Autodesk Inventor part; units mm, degrees
ref_plane "Work Plane1" through (13.4, 0, 0) normal (1, 0, 0) x (0, 1, 0)
ref_plane "XZ Plane" through (0, 0, 0) normal (0, 1, 0) x (-1, 0, 0)
ref_plane "XY Plane" through (0, 0, 0) normal (0, 0, 1) x (1, 0, 0)
sketch "Sketch1" plane through (0, 0, 0) normal (0, 0, 1) x (1, 0, 0)
  circle A0 centre (0, 0) radius 13.4
  circle A1 centre (0, 0) radius 11.75
  dimension "d0" = 26.8
  dimension "d3" = 23.5
extrude "Extrusion1" add sketch "Sketch1" along normal blind 300
ref_plane "Work Plane1" through (13.4, 0, 0) normal (1, 0, 0) x (0, 1, 0)
sketch "Sketch2" plane through (13.4, 0, 0) normal (1, 0, 0) x (0, 1, 0)
  circle A0 centre (0, 30) radius 4
  line L0 (0, -60) -> (0, 360)
  line L1 (13.4, 0) -> (-13.4, 0)
  circle A1 centre (0, 270) radius 4
  line L2 (13.4, 300) -> (-13.4, 300)
  point P0 (0, 0)
  dimension "d4" = 8
  dimension "d5" = 30
  dimension "d6" = 8
  dimension "d7" = 30
extrude "Extrusion2" cut sketch "Sketch2" against normal through all
equation "\"d0\" = PVC_out"
equation "\"d3\" = PVC_in"
equation "\"PVC_out\" = 26.8"
equation "\"PVC_in\" = 23.5"
properties part number "Steering PVC" material "PVC-Piping"
Source: CAD feature listing. Evaluate the final solid. Frame: model axes, mm. Coordinates: 2 decimals unless noted, no trailing zeros. Order: outer loops, then holes, each group sorted by start corner. A loop starts at its lowest first (then second) coordinate and runs counter-clockwise, first axis right, second up.
Item 1: Cut plane A-A (x = 0). Return loops of the section in (y, z), plus the area to 3 significant figures.
Output values:
outline: (-13.4, 0) - (-11.75, 0) - (-11.75, 300) - (-13.4, 300) - close; (11.75, 0) - (13.4, 0) - (13.4, 300) - (11.75, 300) - close
area: 990 mm2
Item 2: Material intervals for line 1 (Z direction, x = 12, y = 0); line 2 (Y direction, x = 0, z = 160); line 3 (Y direction, x = -11.8, z = 270), sorted ascending.
Output values:
line 1: z = 0 to 26, 34 to 266, 274 to 300
line 2: y = -13.4 to -11.75, 11.75 to 13.4
line 3: y = -6.35 to -4, 4 to 6.35
Item 3: Pull-direction query (Y, two-part tool) for faces 1 (the face through (-13.387, -0.589, 147.9)), 2 (the face through (12.24, -0.521, 273.966)), 3 (the face through (0, -12, 0)); classes: pulls with the +Y half, pulls with the -Y half, needs draft (parallel to the pull), parting line crosses it, or undercut.
Output values:
face 1: parting line crosses it
face 2: undercut
face 3: needs draft
Item 4: First-contact query: P1, Ø10, axis at x = -0.5, y = -7.5, coming from the -Z side; P2, Ø6.5, axis at y = 0, z = 270, coming from the +X side; P3, Ø1, axis at y = 8, z = 253, coming from the -X side; P4, Ø1, axis at x = -1.5, z = 158, coming from the -Y side. Flat tips, straight axial feed; report the tip coordinate or a pass-through.
Output values:
P1: stops at z = 0
P2: passes through
P3: stops at x = -11.1
P4: stops at y = -13.36
Item 5: Cut plane B-B (y = 0). Return loops of the section in (x, z), plus the area to 3 significant figures.
Output values:
outline: (-13.4, 0) - (-11.75, 0) - (-11.75, 26) - (-13.4, 26) - close; (-13.4, 34) - (-11.75, 34) - (-11.75, 266) - (-13.4, 266) - close; (-13.4, 274) - (-11.75, 274) - (-11.75, 300) - (-13.4, 300) - close; (11.75, 0) - (13.4, 0) - (13.4, 26) - (11.75, 26) - close; (11.75, 34) - (13.4, 34) - (13.4, 266) - (11.75, 266) - close; (11.75, 274) - (13.4, 274) - (13.4, 300) - (11.75, 300) - close
area: 937 mm2
Item 6: Cut plane D-D (z = 159.5). Return loops of the section in (x, y), plus the area to 3 significant figures.
Output values:
outline: circle Ø26.8 at (0, 0); hole circle Ø23.5 at (0, 0)
area: 130 mm2
Item 7: Cut plane C-C (z = 30). Return loops of the section in (x, y).
Output values:
outline: (-12.79, -4) arc R13.4 ccw to (12.79, -4) - (11.05, -4) arc R11.75 cw to (-11.05, -4) - close; (-12.79, 4) - (-11.05, 4) arc R11.75 cw to (11.05, 4) - (12.79, 4) arc R13.4 ccw to start
